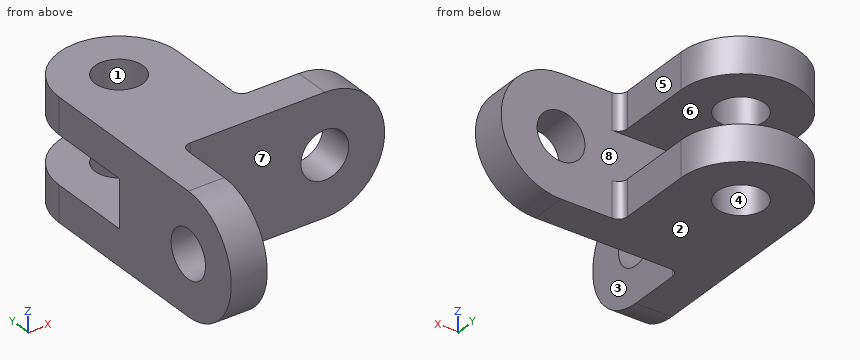
from build123d import *

# Parameters (mm, degrees)
BOSS_EXTRUDE1_DEPTH = 40
BOSS_EXTRUDE2_DEPTH = 12
SKETCH4_R           = 8
CUT_EXTRUDE1_DEPTH  = 12
BOSS_EXTRUDE3_DEPTH = 12
SKETCH6_R           = 8
CUT_EXTRUDE2_DEPTH  = 12
BOSS_EXTRUDE4_DEPTH = 40
SKETCH9_R           = 8
CUT_EXTRUDE3_DEPTH  = 40
SKETCH10_W          = 16
SKETCH10_H          = 52.648113389
CUT_EXTRUDE4_DEPTH  = 62
FILLET1_R           = 3


with BuildPart() as part:
    # Sketch1 → Boss-Extrude1 (new body)
    with BuildSketch(Plane.XY):
        Polygon((-46.523076923, -20), (-34.523076923, -20), (-34.523076923, 0), (13.476923077, 0), (13.476923077, 12), (-6.523076923, 12), (-6.523076923, 40), (-46.523076923, 40), align=None)
    extrude(amount=BOSS_EXTRUDE1_DEPTH)

    # Sketch3 → Boss-Extrude2 (add)
    with BuildSketch(Plane(origin=(-34.523076923, 0, 0), x_dir=(0, 0, -1), z_dir=(1, 0, 0))):
        with BuildLine():
            Line((-40, -20), (0, -20))
            ThreePointArc((0, -20), (-20, -40), (-40, -20))
        make_face()
    extrude(amount=-BOSS_EXTRUDE2_DEPTH)

    # Sketch4 → Cut-Extrude1 (cut)
    with BuildSketch(Plane(origin=(-34.523076923, 0, 0), x_dir=(0, 0, -1), z_dir=(1, 0, 0))):
        with Locations((-20, -20)):
            Circle(SKETCH4_R)
    extrude(amount=-CUT_EXTRUDE1_DEPTH, mode=Mode.SUBTRACT)

    # Sketch5 → Boss-Extrude3 (add)
    with BuildSketch(Plane(origin=(0, 12, 0), x_dir=(1, 0, 0), z_dir=(0, 1, 0))):
        with BuildLine():
            Line((13.476923077, 0), (13.476923077, -40))
            ThreePointArc((13.476923077, -40), (33.476923077, -20), (13.476923077, 0))
        make_face()
    extrude(amount=-BOSS_EXTRUDE3_DEPTH)

    # Sketch6 → Cut-Extrude2 (cut)
    with BuildSketch(Plane(origin=(0, 12, 0), x_dir=(1, 0, 0), z_dir=(0, 1, 0))):
        with Locations(Location((13.476923077, -20, 0), (0, 0, 180))):
            Circle(SKETCH6_R)
    extrude(amount=-CUT_EXTRUDE2_DEPTH, mode=Mode.SUBTRACT)

    # Sketch8 → Boss-Extrude4 (add)
    with BuildSketch(Plane.XY.offset(40)):
        with BuildLine():
            Line((-46.523076923, 40), (-6.523076923, 40))
            ThreePointArc((-6.523076923, 40), (-26.523076923, 60), (-46.523076923, 40))
        make_face()
    extrude(amount=-BOSS_EXTRUDE4_DEPTH)

    # Sketch9 → Cut-Extrude3 (cut)
    with BuildSketch(Plane.XY.offset(40)):
        with Locations((-26.523076923, 40)):
            Circle(SKETCH9_R)
    extrude(amount=-CUT_EXTRUDE3_DEPTH, mode=Mode.SUBTRACT)

    # Sketch10 → Cut-Extrude4 (cut)
    with BuildSketch(Plane(origin=(-6.523076923, 0, 0), x_dir=(0, 0, -1), z_dir=(1, 0, 0))):
        with Locations((-20, 38.324056695)):
            Rectangle(SKETCH10_W, SKETCH10_H)
    extrude(amount=-CUT_EXTRUDE4_DEPTH, mode=Mode.SUBTRACT)

    # Fillet1
    fillet1_edges = [part.edges().sort_by_distance(p)[0] for p in [
        (-6.523076923, 12, 34),
        (-34.523076923, 0, 20),
        (-6.523076923, 12, 6),
    ]]
    fillet(fillet1_edges, radius=FILLET1_R)


solid = part.part
Geometry: final body of the model. Coordinates: model frame, mm. Face numbers are marked on the shaded views. A direction names the side the tool comes from. Coordinates: 2 decimals unless noted, no trailing zeros. Order: outer loops, then holes, each group sorted by start corner. A loop starts at its lowest first (then second) coordinate and runs counter-clockwise, first axis right, second up.
(1) First-contact query: pin 1 (12 mm diameter, centred on x = 24, z = 30.5, fed in from +Y); pin 2 (6 mm diameter, centred on y = 25, z = 35.5, fed in from +X); pin 3 (1.5 mm diameter, centred on y = -22, z = 15, fed in from -X); pin 4 (1 mm diameter, centred on y = -10, z = 22.5, fed in from +X). Flat tips, straight axial feed; report the tip coordinate or a pass-through.
(2) Draft query along X for the marked faces 1, 2, 3 and 4. Return one class per face: pulls with the +X half, pulls with the -X half, needs draft (parallel to the pull), parting line crosses it, or undercut.
(3) Section query C-C (x = 20). Return the cut outline in (y, z).
(4) Section query A-A (z = 20). Return the cut outline in (x, y), plus the area to 3 significant figures.
(5) Access query for the marked faces 5, 6, 7 and 8. Directions: +Z, -Z, +X, -X, +Y, -Y. A direction counts if a zero-diameter tool reaches every point of the face in a straight line with its end or side. Return the directions, or none.
(6) Section query B-B (y = 23). Return the cut outline in (x, z), plus the area to 3 significant figures.
(7) Material intervals for probe 1 along Z at (x, y) = (-21, 54); probe 2 along Y at (x, z) = (21, 9); probe 3 along X at (y, z) = (42.5, 3), sorted ascending.
(8) Section query D-D (y = 45.5). Return the cut outline in (x, z).
Solution:
1. pin 1: stops at y = 12
1. pin 2: stops at x = -6.52
1. pin 3: passes through
1. pin 4: stops at x = -34.52
2. face 1: undercut
2. face 2: needs draft
2. face 3: pulls with the +X half
2. face 4: undercut
3. outline: (0, 1.09) - (12, 1.09) - (12, 15.37) - (0, 15.37) - close; (0, 24.63) - (12, 24.63) - (12, 38.91) - (0, 38.91) - close
4. outline: (-46.52, -40) - (-34.52, -40) - (-34.52, -28) - (-46.52, -28) - close; (-46.52, -12) - (-34.52, -12) - (-34.52, -3) arc R3 cw to (-31.52, 0) - (5.48, 0) - (5.48, 12) - (-46.52, 12) - close; (21.48, 0) - (33.48, 0) - (33.48, 12) - (21.48, 12) - close
4. area: 1,060 mm2
5. face 5: +Z, -Z, +X, +Y
5. face 6: +X, -X, +Y
5. face 7: +Z, -Z, +X, -Y
5. face 8: +X, +Y
6. outline: (-46.52, 0) - (-6.52, 0) - (-6.52, 12) - (-46.52, 12) - close; (-46.52, 28) - (-6.52, 28) - (-6.52, 40) - (-46.52, 40) - close
6. area: 960 mm2
7. probe 1: z = 0 to 12, 28 to 40
7. probe 2: y = 0 to 12
7. probe 3: x = -46.37 to -34.12, -18.92 to -6.68
8. outline: (-45.75, 0) - (-32.33, 0) - (-32.33, 12) - (-45.75, 12) - close; (-45.75, 28) - (-32.33, 28) - (-32.33, 40) - (-45.75, 40) - close; (-20.71, 0) - (-7.29, 0) - (-7.29, 12) - (-20.71, 12) - close; (-20.71, 28) - (-7.29, 28) - (-7.29, 40) - (-20.71, 40) - close
